Input: part model. Units: mm. Frame: model coordinates. Face numbers are marked on the shaded views. Coordinates: 2 decimals unless noted, no trailing zeros. Write each loop counter-clockwise with the first axis right and the second up, starting at its lowest first coordinate (ties: lowest second). Pieces come first, ordered by that corner, then holes. Notation, with made-up numbers: M -29,65 L 27,65 A29 cw 27,97 Z; hole C 5.25,27 d8. An arc over 180 degrees is marked long. Use one line per item in the form item = value.
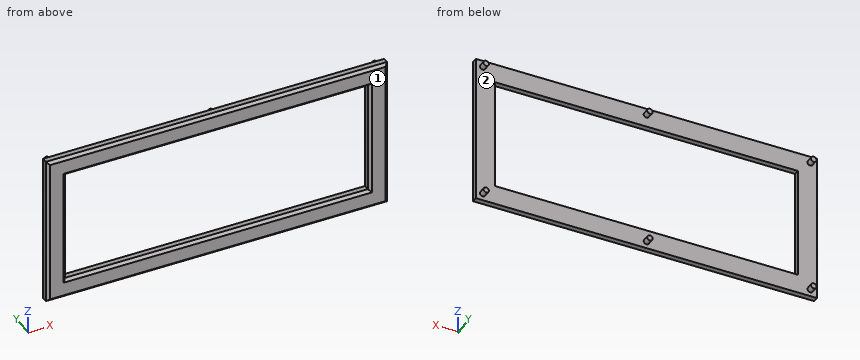
from build123d import *

# Parameters (mm, degrees)
F0_W     = 125
F0_H     = 55
F0_W_2   = 111
F0_H_2   = 41
F1_DEPTH = 3
F2_R     = 1
F3_DEPTH = 2.5
F4_SIZE  = 1


with BuildPart() as f1:
    # F0 (on Front) → F1 (new body)
    with BuildSketch(Plane.XZ):
        with Locations((62.5, 27.5)):
            Rectangle(F0_W, F0_H)
        with Locations((62.5, 27.5)):
            Rectangle(F0_W_2, F0_H_2, mode=Mode.SUBTRACT)
    extrude(amount=F1_DEPTH)

    # F2 (on face) → F3 (join)
    with BuildSketch(Plane(origin=(0, 0, 0), x_dir=(-1, 0, 0), z_dir=(0, 1, 0))):
        with Locations((-2.5, 52.5)):
            Circle(F2_R)
        with Locations((-62.5, 2.5)):
            Circle(F2_R)
        with Locations((-122.5, 52.5)):
            Circle(F2_R)
        with Locations((-122.5, 2.5)):
            Circle(F2_R)
        with Locations((-62.5, 52.5)):
            Circle(F2_R)
        with Locations((-2.5, 2.5)):
            Circle(F2_R)
    extrude(amount=F3_DEPTH)

    # F4
    f4_edges = [f1.edges().sort_by_distance(p)[0] for p in [
        (0, -3, 27.5),
        (62.5, -3, 0),
        (125, -3, 27.5),
        (62.5, -3, 55),
        (62.5, -3, 48),
        (118, -3, 27.5),
        (62.5, -3, 7),
        (7, -3, 27.5),
    ]]
    chamfer(f4_edges, length=F4_SIZE)


solid = f1.part
(1) Line query: probe 1 along X at (y, z) = (-1.95, 9); probe 2 along Z at (x, y) = (72, -1.7); probe 3 along Y at (x, z) = (105.5, 49.5). Output: solid intervals per line, ascending.
Computed:
probe_1 = 0 to 7, 118 to 125
probe_2 = 0 to 7, 48 to 55
probe_3 = -3 to 0
(2) First-contact query: pin 1 Ø2 at (y, z) = (-2.5, 30.5) entering from +X; pin 2 Ø1.5 at (x, y) = (105, 1) entering from -Z. Flat tips, straight axial feed; report the tip coordinate or a pass-through.
Computed:
pin_1 = 125
pin_2 = through
(3) Section query B-B on x = 12.5. Return the cut outline in (y, z), plus the area to 3 significant figures.
Computed:
outline = M -3,1 L -2,0 L 0,0 L 0,7 L -2,7 L -3,6 Z; M -3,49 L -2,48 L 0,48 L 0,55 L -2,55 L -3,54 Z
area = 40.0 mm^2
(4) Pull-direction query (X, two-part tool) for the marked faces 1 and 2; classes: pulls with the +X half, pulls with the -X half, needs draft (parallel to the pull), parting line crosses it, or undercut.
Computed:
face_1 = needs draft
face_2 = undercut
(5) Section query A-A on z = 10. Return the cut outline in (x, y), plus the area to 3 significant figures.
Computed:
outline = M 0,-2 L 1,-3 L 6,-3 L 7,-2 L 7,0 L 0,0 Z; M 118,-2 L 119,-3 L 124,-3 L 125,-2 L 125,0 L 118,0 Z
area = 40.0 mm^2
